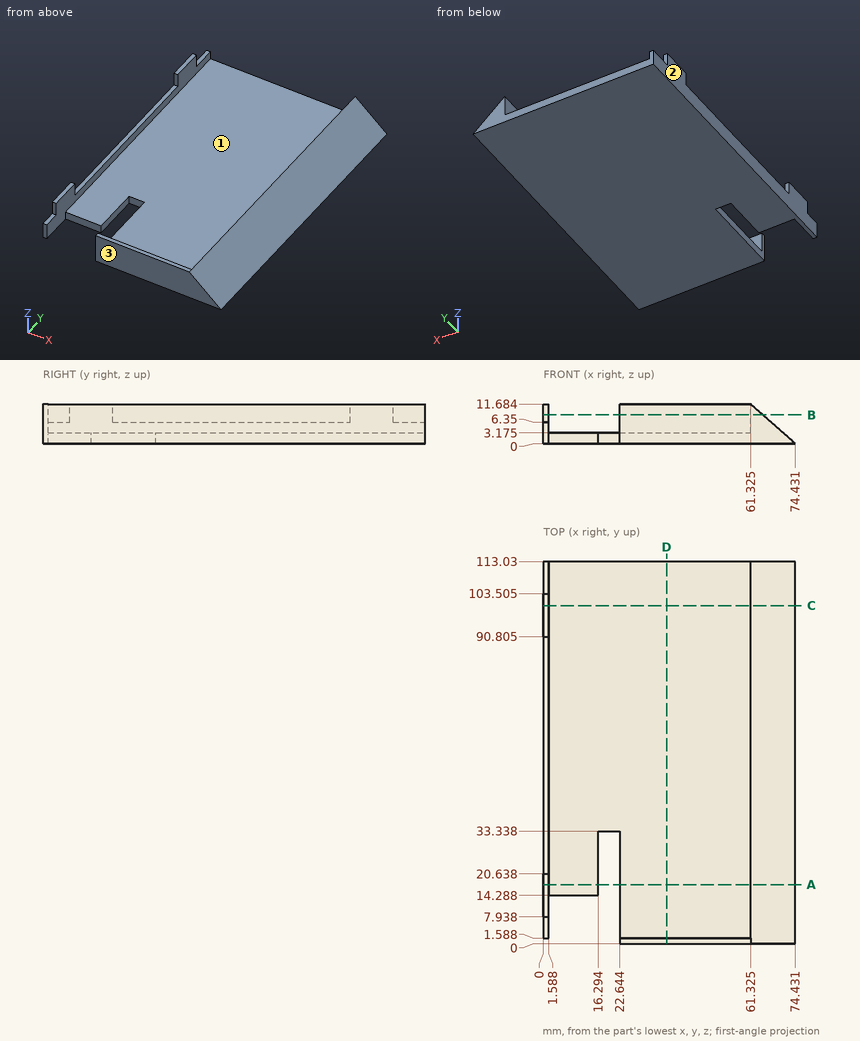
Design review of the part shown in the three views and the two pictorial views. Dimensions are in mm from the part's minimum x, y and z. Coordinates: 2 decimals unless noted, no trailing zeros. Loops run counter-clockwise (first coordinate to the right, second up) from the corner with the lowest first, then second, coordinate; pieces in that order, holes last.
(1) Consider section D-D, the plane x = 36.5. Give the boundary of the cut face in (y, z) (1 decimal).
Determined:
outline: (0, 0) - (113, 0) - (113, 3.2) - (1.6, 3.2) - (1.6, 11.7) - (0, 11.7) - close
(2) Wall thickness on L1, parallel to Y at x = 34.5, z = 8; L2, parallel to Y at x = 3.5, z = 3; L3, parallel to X at y = 101, z = 5.75 (1 decimal): over which ranges is each line inside the solid? List them lowest first.
Determined:
L1: y = 0 to 1.59
L2: y = 14.29 to 113.03
L3: x = 0 to 1.6, 61.3 to 68
(3) Consider section B-B, the plane z = 8.5. Give the boundary of the cut face in (x, y) (1 decimal).
Determined:
outline: (0, 7.9) - (1.6, 7.9) - (1.6, 20.6) - (0, 20.6) - close; (0, 90.8) - (1.6, 90.8) - (1.6, 103.5) - (0, 103.5) - close; (22.6, 0) - (64.9, 0) - (64.9, 113) - (61.3, 113) - (61.3, 1.6) - (22.6, 1.6) - close
(4) Consider section C-C, the plane y = 100. Give the boundary of the cut face in (x, z) (1 decimal), plus the area to 3 significant figures.
Determined:
outline: (0, 0) - (74.4, 0) - (61.3, 11.7) - (61.3, 3.2) - (1.6, 3.2) - (1.6, 11.7) - (0, 11.7) - close
area: 285 mm2
(5) Consider section A-A, the plane y = 17.5. Give the boundary of the cut face in (x, z) (1 decimal).
Determined:
outline: (0, 0) - (16.3, 0) - (16.3, 3.2) - (1.6, 3.2) - (1.6, 11.7) - (0, 11.7) - close; (22.6, 0) - (74.4, 0) - (61.3, 11.7) - (61.3, 3.2) - (22.6, 3.2) - close
(6) Insertion check: P1, Ø2.5, axis at x = 20.5, z = 2, coming from the -Y side; P2, Ø1.3, axis at x = 1, z = 10.5, coming from the -Y side; P3, Ø1.7, axis at x = 1, y = 4, coming from the +Z side; P4, Ø2, axis at x = 67, z = 9, coming from the -Y side. Each pin has a flat end and moves straight along its axis. Give the tip position at first contact, or say it passes through.
Determined:
P1: stops at y = 33.34
P2: stops at y = 7.94
P3: stops at z = 6.35
P4: passes through
(7) Draft analysis for pull direction X (two halves, no side actions). For the marked faces 1, 2 and 3, state which applies: +X half, -X half, draft (parallel to the pull), parting line (faces both ways), or undercut.
Determined:
face 1: undercut
face 2: -X half
face 3: draft
